Source: CAD feature listing. Evaluate the final solid. Frame: model axes, mm. A direction names the side the tool comes from. Round coordinates to 2 decimals unless told otherwise and drop trailing zeros. Order: outer loops, then holes, each group sorted by start corner. A loop starts at its lowest first (then second) coordinate and runs counter-clockwise, first axis right, second up. Notation, with made-up numbers: (-9, 61) - (49, 61) arc R26 ccw to (49, 88) - close; hole circle Ø2 at (16, 22.25). An arc over 180 degrees is marked (long way). Put each result on its own line as item: value. Start each with the question number.
1) Section B-B on x = 16. Output: boundary loops of the cut face in (y, z).
2) Contact query for flat-ended pins moving along their axis: P1, Ø4, axis at y = 8.5, z = 10, coming from the +X side; P2, Ø3, axis at y = 2.5, z = 11.5, coming from the +X side; P3, Ø2, axis at x = 3.5, y = 3, coming from the +Z side. Output: stop coordinate, or through.
3) Section A-A on z = 0. Output: boundary loops of the cut face in (x, y) (3 decimals).
4) Mould query, pull axis Z, two halves, no side actions, for faces 3 (the face through (-22, 5, -14)), 4 (the face through (-6, 8, 6)), 5 (the face through (6.52, 2.54, 29.36)), 6 (the face through (1.669, 6.226, 7.517)). Classes: +Z half, -Z half, draft (parallel to the pull), parting line (faces both ways), or undercut.
5) Section C-C on x = -13. Output: boundary loops of the cut face in (y, z), then the cut area to 3 significant figures.
6) Access query for faces 1 (the face through (0, 0, 0)), 2 (the face through (-13.86, 7.54, -21.73)). Directions: +Z, -Z, +X, -X, +Y, -Y. A direction counts if a zero-diameter tool reaches every point of the face in a straight line with its end or side. Return the directions, or none.
7) Section D-D on z = -17. Output: boundary loops of the cut face in (x, y), then the cut area to 3 significant figures.
8) Line query: probe 1 along Z at (x, y) = (0, 6.9) (3 decimals); probe 2 along X at (y, z) = (6, 0) (3 decimals); probe 3 along Z at (x, y) = (0, 8.55) (3 decimals). Output: solid intervals per line, ascending. Write a range as [from, to].
```python
from build123d import *

# Parameters (mm, degrees)
SKETCH2_R          = 3.5
CUT_EXTRUDE1_DEPTH = 10
SKETCH3_R          = 0.5
CUT_EXTRUDE2_DEPTH = 5


with BuildPart() as part:
    # Sketch1 → Revolve1 (revolve)
    with BuildSketch(Plane.XY):
        Polygon((0, 0), (-30.075, 0), (-30.075, 5), (-25.775, 5), (-25.775, 10), (-13.7, 10), (-13.7, 8), (-7.7, 8), (-7.7, 4.5), (0, 4.5), align=None)
    revolve(axis=Axis((0, 4.5, 0), (0, -1, 0)))

    # Sketch2 → Cut-Extrude1 (cut)
    with BuildSketch(Plane(origin=(0, 10, 0), x_dir=(1, 0, 0), z_dir=(0, 1, 0))):
        with Locations((15.8, 0)):
            Circle(SKETCH2_R)
    extrude(amount=-CUT_EXTRUDE1_DEPTH, mode=Mode.SUBTRACT)

    # Sketch3 → Cut-Extrude2 (cut, symmetric)
    with BuildSketch(Plane(origin=(0, 5, 0), x_dir=(1, 0, 0), z_dir=(0, 1, 0))):
        with Locations((0, 23.625)):
            Circle(SKETCH3_R)
    extrude(amount=CUT_EXTRUDE2_DEPTH, both=True, mode=Mode.SUBTRACT)


solid = part.part
```
Answer sheet:
1. outline: (0, -25.47) - (5, -25.47) - (5, -20.21) - (10, -20.21) - (10, -3.49) - (0, -3.49) - close; (0, 3.49) - (10, 3.49) - (10, 20.21) - (5, 20.21) - (5, 25.47) - (0, 25.47) - close
2. P1: x = 24.5
2. P2: x = 28.36
2. P3: z = 29.97
3. outline: (-30.075, 0) - (12.3, 0) - (12.3, 8) - (7.7, 8) - (7.7, 4.5) - (-7.7, 4.5) - (-7.7, 8) - (-13.7, 8) - (-13.7, 10) - (-25.775, 10) - (-25.775, 5) - (-30.075, 5) - close; (19.3, 0) - (30.075, 0) - (30.075, 5) - (25.775, 5) - (25.775, 10) - (19.3, 10) - close
4. face 3: draft
4. face 4: undercut
4. face 5: parting line
4. face 6: undercut
5. outline: (0, -27.12) - (5, -27.12) - (5, -22.26) - (10, -22.26) - (10, -4.32) - (8, -4.32) - (8, 4.32) - (10, 4.32) - (10, 22.26) - (5, 22.26) - (5, 27.12) - (0, 27.12) - close
5. area: 476 mm^2
6. face 1: +Z, -Z, +X, -X, -Y
6. face 2: +Y
7. outline: (-24.81, 0) - (24.81, 0) - (24.81, 5) - (19.37, 5) - (19.37, 10) - (-19.37, 10) - (-19.37, 5) - (-24.81, 5) - close
7. area: 442 mm^2
8. probe 1: [-25.775, -24.125], [-23.125, -7.7], [7.7, 25.775]
8. probe 2: [-25.775, -7.7], [7.7, 12.3], [19.3, 25.775]
8. probe 3: [-25.775, -24.125], [-23.125, -13.7], [13.7, 25.775]
